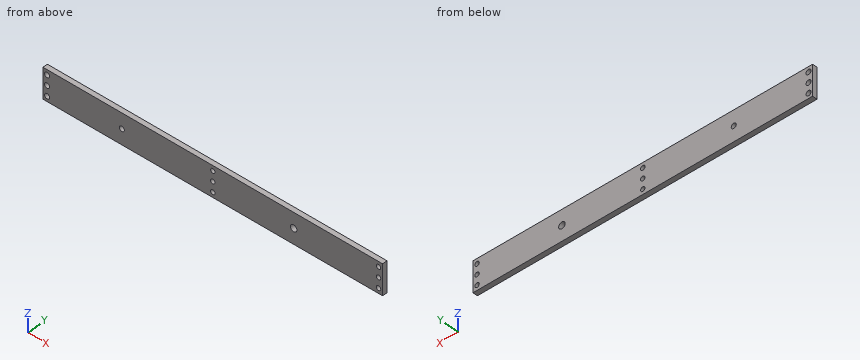
```python
from build123d import *

# Parameters (mm, degrees)
ESBO_O1_R                = 2.5
ESBO_O1_R_2              = 2.2
ESBO_O1_R_3              = 3.225
ESBO_O1_W                = 8
ESBO_O1_H                = 30
RESSALTO_EXTRUS_O1_DEPTH = 4.7625


with BuildPart() as part:
    # Esboço1 → Ressalto-extrusão1 (new body)
    # profile 1 of 2: a face of its own
    with BuildSketch(Plane(origin=(0, 0, 0), x_dir=(1, 0, 0), z_dir=(0, 1, 0))):
        Polygon((-160, -15), (160, -15), (160, 15), (-160, 15), (-168, 15), (-168, -15), align=None)
        with Locations(Location((-164, -10, 0), (0, 0, 90))):
            Circle(ESBO_O1_R, mode=Mode.SUBTRACT)
        with Locations(Location((0, -10, 0), (0, 0, 90))):
            Circle(ESBO_O1_R_2, mode=Mode.SUBTRACT)
        with Locations(Location((-164, 0, 0), (0, 0, 90))):
            Circle(ESBO_O1_R, mode=Mode.SUBTRACT)
        with Locations(Location((-90, 0, 0), (0, 0, 90))):
            Circle(ESBO_O1_R, mode=Mode.SUBTRACT)
        with Locations(Location((-164, 10, 0), (0, 0, 90))):
            Circle(ESBO_O1_R, mode=Mode.SUBTRACT)
        with Locations(Location((0, 0, 0), (0, 0, 90))):
            Circle(ESBO_O1_R_2, mode=Mode.SUBTRACT)
        with Locations(Location((80, 0, 0), (0, 0, 90))):
            Circle(ESBO_O1_R_3, mode=Mode.SUBTRACT)
        with Locations(Location((0, 10, 0), (0, 0, 90))):
            Circle(ESBO_O1_R_2, mode=Mode.SUBTRACT)
    # profile 2 of 2: a face of its own
    with BuildSketch(Plane(origin=(0, 0, 0), x_dir=(1, 0, 0), z_dir=(0, 1, 0))):
        with Locations((164, 0)):
            Rectangle(ESBO_O1_W, ESBO_O1_H)
        with Locations(Location((164, -10, 0), (0, 0, 90))):
            Circle(ESBO_O1_R_2, mode=Mode.SUBTRACT)
        with Locations(Location((164, 0, 0), (0, 0, 90))):
            Circle(ESBO_O1_R_2, mode=Mode.SUBTRACT)
        with Locations(Location((164, 10, 0), (0, 0, 90))):
            Circle(ESBO_O1_R_2, mode=Mode.SUBTRACT)
    extrude(amount=RESSALTO_EXTRUS_O1_DEPTH)


solid = part.part
```
Design review of the part built by this model. Coordinates are the model's own, in mm. Round coordinates to 2 decimals unless told otherwise and drop trailing zeros. Write each loop counter-clockwise with the first axis right and the second up, starting at its lowest first coordinate (ties: lowest second). Pieces come first, ordered by that corner, then holes. Notation, with made-up numbers: (-26, 43) -> (7, 43) arc R12 cw to (7, 57) -> close; hole circle Ø9 at (19, -22). An arc over 180 degrees is marked (long way). Write item = value, one per line. Start each with the question number.
1) Take a section at A-A, the plane x = 80. State the section outline as (y, z) points (1 decimal).
2) Take a section at B-B, the plane y = 2.3. Count the separate pieces of the cut face and the enclosed holes in it, plus the area to 3 significant figures.
3) Wall thickness on probe 1 along Z at (x, y) = (164, 1.35); probe 2 along X at (y, z) = (1.7, 0) (3 decimals); probe 3 along X at (y, z) = (3.5, 10): over which ranges is each line inside the solid? List them lowest first. Write a range as from..to.
Results list:
q1.outline = (0, -15) -> (4.8, -15) -> (4.8, -3.2) -> (0, -3.2) -> close; (0, 3.2) -> (4.8, 3.2) -> (4.8, 15) -> (0, 15) -> close
q2.separate_pieces = 1
q2.enclosed_holes = 11
q2.area = 9,880 mm²
q3.probe_1 = -15..-12.2, -7.8..-2.2, 2.2..7.8, 12.2..15
q3.probe_2 = -168..-166.5, -161.5..-92.5, -87.5..-2.2, 2.2..76.775, 83.225..161.8, 166.2..168
q3.probe_3 = -168..-166.5, -161.5..-2.2, 2.2..161.8, 166.2..168
